Part print with two shaded views. Sizes in mm from the minimum x, y, z corner. Coordinates: 2 decimals unless noted, no trailing zeros. Loops run counter-clockwise (first coordinate to the right, second up) from the corner with the lowest first, then second, coordinate; pieces in that order, holes last.
Item 1: Cut at A-A (y = 4). List the corners of the cut face in (x, z).
Item 2: Flat gauge pins, fed straight in: pin 1 (2 mm diameter, centred on y = 2, z = 36.5, fed in from +X); pin 2 (1.5 mm diameter, centred on y = 4, z = 17, fed in from +X); pin 3 (2 mm diameter, centred on x = 5.5, z = 12, fed in from +Y). Where does each tip first touch, or does it go through?
Item 3: Cut at C-C (x = 6.75). List the corners of the cut face in (y, z).
Item 4: Mould opens along Z. For the marked faces 1, 2 and 3 say: released by +Z, released by -Z, zero draft, split by the parting line, or undercut.
Item 5: Cut at D-D (z = 37). List the corners of the cut face in (x, y).
Item 6: Drill centre lines: line 1 along Z through (x, y) = (5.5, 7.25); line 2 along Y through (x, z) = (5.5, 35); line 3 along X through (y, z) = (3.75, 11.5). Where is each one in solid material? Low to high.
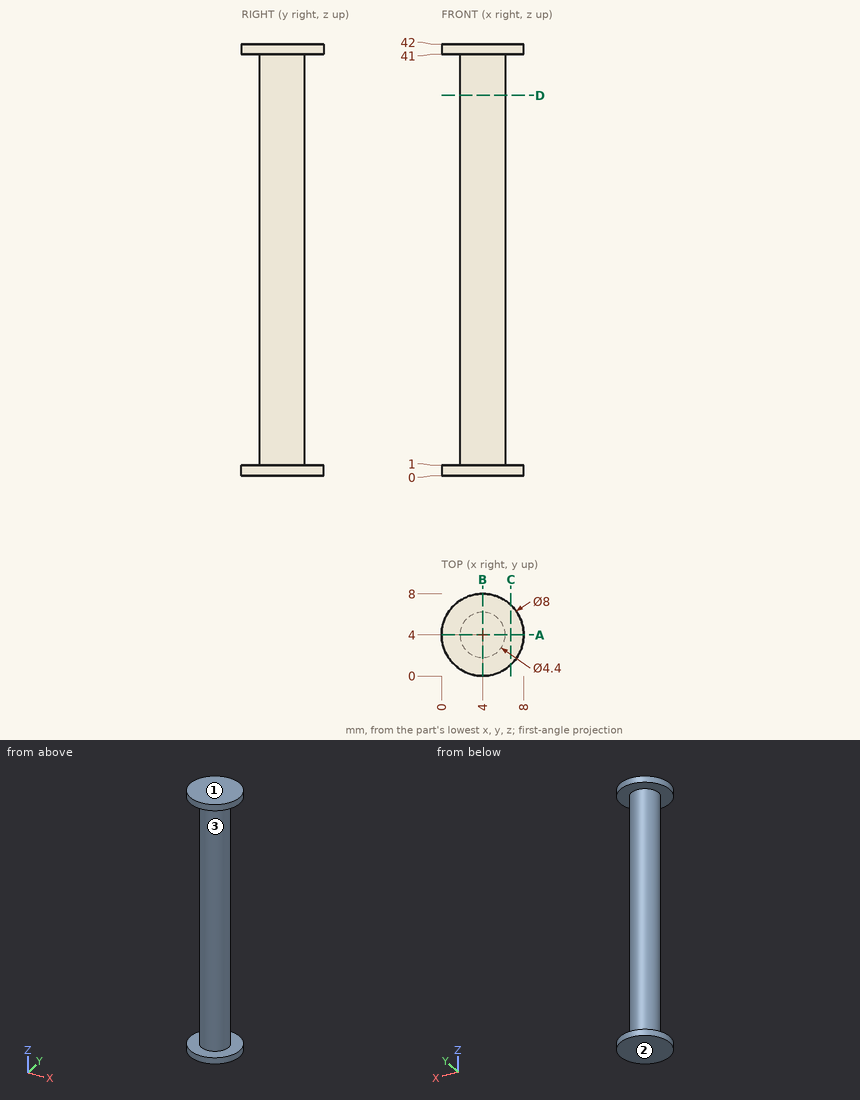
Filled sheet:
1. outline: (0, 0) - (8, 0) - (8, 1) - (6.2, 1) - (6.2, 41) - (8, 41) - (8, 42) - (0, 42) - (0, 41) - (1.8, 41) - (1.8, 1) - (0, 1) - close
2. pin 1: stops at x = 5.96
2. pin 2: stops at x = 6.2
2. pin 3: stops at y = 6.14
3. outline: (1.1, 0) - (6.9, 0) - (6.9, 1) - (1.1, 1) - close; (1.1, 41) - (6.9, 41) - (6.9, 42) - (1.1, 42) - close
4. face 1: released by +Z
4. face 2: released by -Z
4. face 3: undercut
5. outline: circle Ø4.4 at (4, 4)
6. line 1: z = 0 to 1, 41 to 42
6. line 2: y = 2.39 to 5.61
6. line 3: x = 1.81 to 6.19
